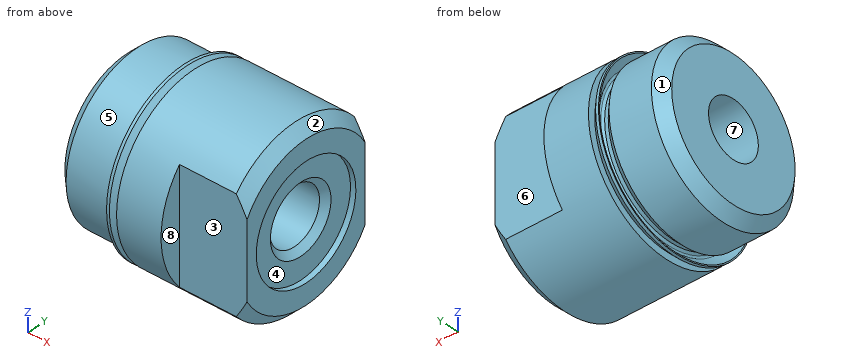
Autodesk Inventor part; units mm, degrees
ref_plane "cut1_XY" through (12.7, 4.699, 0) normal (1, 0, 0) x (0, 0, -1)
ref_plane "cut1_YZ" through (12.7, 4.699, 0) normal (0, 0, -1) x (0, 1, 0)
ref_plane "cut1_ZX" through (12.7, 4.699, 0) normal (0, 1, 0) x (1, 0, 0)
sketch "Sketch_1" plane through (0, 0, 0) normal (0, 0, 1) x (1, 0, 0)
  line L0 (12.7, 0) -> (0, 0)
  line L1 (0, 0) -> (0, 4.9085)
  line L2 (0, 4.9085) -> (0.762, 5.6706)
  line L3 (0.762, 5.6706) -> (3.7592, 5.6706)
  line L4 (3.7592, 5.6706) -> (4.2672, 5.1626)
  line L5 (4.2672, 5.1626) -> (4.7752, 5.1626)
  line L6 (4.7752, 5.1626) -> (4.7752, 6.1659)
  line L7 (4.7752, 6.1659) -> (11.938, 6.1659)
  line L8 (11.938, 6.1659) -> (12.7, 5.4039)
  line L9 (12.7, 5.4039) -> (12.7, 0)
  line L10 (12.7, 0) -> (0, 0)
revolve "Revolution1" add sketch "Sketch_1" angle 360 about axis through (12.7, 0, 0) along (1, 0, 0)
sketch "Sketch2" plane through (12.7, 0, 0) normal (1, 0, 0) x (0, 0, -1)
  point P0 (0, 0)
hole "Hole1" at (12.7, 0, 0) direction (-1, 0, 0) diameter 7.9248 depth 0.381
sketch "Sketch3" plane through (12.319, 0, 0) normal (1, 0, 0) x (0, 0, -1)
  point P0 (0, 0)
hole "Hole2" at (12.319, 0, 0) direction (-1, 0, 0) diameter 3.9624 depth 12.319 countersink diameter 4.826 countersink angle 90
sketch "Sketch_5" plane through (12.7, 0, 0) normal (1, 0, 0) x (0, 0, -1)
  line L0 (-24.6634, -12.3317) -> (24.6634, -12.3317)
  line L1 (24.6634, -12.3317) -> (24.6634, 12.3317)
  line L2 (24.6634, 12.3317) -> (-24.6634, 12.3317)
  line L3 (-24.6634, 12.3317) -> (-24.6634, -12.3317)
  line L4 (-12.3317, -4.699) -> (12.3317, -4.699)
  line L5 (12.3317, -4.699) -> (12.3317, 4.699)
  line L6 (12.3317, 4.699) -> (-12.3317, 4.699)
  line L7 (-12.3317, 4.699) -> (-12.3317, -4.699)
extrude "Extrusion1" cut sketch "Sketch_5" against normal blind 4.7752
sketch "Sketch_24" plane through (0, 0, 0) normal (0, 0, 1) x (1, 0, 0)
  line L0 (4.7752, 0) -> (4.2672, 0)
  line L1 (4.0665, 6.1659) -> (4.0665, 6.0817)
  line L2 (4.0665, 6.0817) -> (4.6636, 5.4846)
  arc A0 (4.6636, 5.305) -> (4.6636, 5.4846) centre (4.5738, 5.3948) ccw
  line L3 (4.6636, 5.305) -> (4.5212, 5.1626)
  line L4 (4.5212, 5.1626) -> (4.2672, 5.1626)
  line L5 (4.2672, 5.1626) -> (4.2672, 4.9085)
  line L6 (4.2672, 4.9085) -> (4.7752, 4.9085)
  line L7 (4.7752, 4.9085) -> (4.7752, 5.6603)
  line L8 (4.7752, 5.6603) -> (4.2697, 6.1659)
  line L9 (4.2697, 6.1659) -> (4.0665, 6.1659)
revolve "Revolution2" add sketch "Sketch_24" angle 360 about axis through (4.7752, 0, 0) along (1, 0, 0)
ref_plane "cut1_XY" through (12.7, 4.699, 0) normal (1, 0, 0) x (0, 0, -1)
ref_plane "cut1_YZ" through (12.7, 4.699, 0) normal (0, 0, -1) x (0, 1, 0)
ref_plane "cut1_ZX" through (12.7, 4.699, 0) normal (0, 1, 0) x (1, 0, 0)
ref_plane "cut2_XY" through (12.7, -4.699, 0) normal (1, 0, 0) x (0, 0, -1)
ref_plane "cut2_YZ" through (12.7, -4.699, 0) normal (0, 0, -1) x (0, 1, 0)
ref_plane "cut2_ZX" through (12.7, -4.699, 0) normal (0, 1, 0) x (1, 0, 0)
ref_plane "cutf1_XY" through (12.7, 0, 0) normal (0, 0, 1) x (1, 0, 0)
ref_plane "cutf1_YZ" through (12.7, 0, 0) normal (1, 0, 0) x (0, 1, 0)
ref_plane "cutf1_ZX" through (12.7, 0, 0) normal (0, 1, 0) x (0, 0, 1)
ref_plane "cutf2_XY" through (7.9248, 0, 0) normal (0, 0, 1) x (1, 0, 0)
ref_plane "cutf2_YZ" through (7.9248, 0, 0) normal (1, 0, 0) x (0, 1, 0)
ref_plane "cutf2_ZX" through (7.9248, 0, 0) normal (0, 1, 0) x (0, 0, 1)
ref_plane "lovra_XY" through (12.7, 0, 0) normal (1, 0, 0) x (0, 1, 0)
ref_plane "lovra_YZ" through (12.7, 0, 0) normal (0, 1, 0) x (0, 0, 1)
ref_plane "lovra_ZX" through (12.7, 0, 0) normal (0, 0, 1) x (1, 0, 0)
ref_plane "lovra1_XY" through (7.9248, 0, 0) normal (1, 0, 0) x (0, 0, -1)
ref_plane "lovra1_YZ" through (7.9248, 0, 0) normal (0, 0, -1) x (0, 1, 0)
ref_plane "lovra1_ZX" through (7.9248, 0, 0) normal (0, 1, 0) x (1, 0, 0)
ref_plane "lovra2_XY" through (7.9248, 4.699, 0) normal (1, 0, 0) x (0, 0, -1)
ref_plane "lovra2_YZ" through (7.9248, 4.699, 0) normal (0, 0, -1) x (0, 1, 0)
ref_plane "lovra2_ZX" through (7.9248, 4.699, 0) normal (0, 1, 0) x (1, 0, 0)
ref_plane "lovra21_XY" through (0, 0, 5.2705) normal (1, 0, 0) x (0, 0, -1)
ref_plane "lovra21_YZ" through (0, 0, 5.2705) normal (0, 0, -1) x (0, 1, 0)
ref_plane "lovra21_ZX" through (0, 0, 5.2705) normal (0, 1, 0) x (1, 0, 0)
ref_plane "lovra22_XY" through (0, 0, -5.2705) normal (1, 0, 0) x (0, 0, -1)
ref_plane "lovra22_YZ" through (0, 0, -5.2705) normal (0, 0, -1) x (0, 1, 0)
ref_plane "lovra22_ZX" through (0, 0, -5.2705) normal (0, 1, 0) x (1, 0, 0)
ref_plane "lovra3_XY" through (7.9248, -4.699, 0) normal (1, 0, 0) x (0, 0, -1)
ref_plane "lovra3_YZ" through (7.9248, -4.699, 0) normal (0, 0, -1) x (0, 1, 0)
ref_plane "lovra3_ZX" through (7.9248, -4.699, 0) normal (0, 1, 0) x (1, 0, 0)
ref_plane "olen_XY" through (12.7, 0, 0) normal (1, 0, 0) x (0, 0, -1)
ref_plane "olen_YZ" through (12.7, 0, 0) normal (0, 0, -1) x (0, 1, 0)
ref_plane "olen_ZX" through (12.7, 0, 0) normal (0, 1, 0) x (1, 0, 0)
ref_plane "to_mounting_bracket_XY" through (17.4752, 0, 0) normal (1, 0, 0) x (0, 0, -1)
ref_plane "to_mounting_bracket_YZ" through (17.4752, 0, 0) normal (0, 0, -1) x (0, 1, 0)
ref_plane "to_mounting_bracket_ZX" through (17.4752, 0, 0) normal (0, 1, 0) x (1, 0, 0)
ref_plane "to_nut_XY" through (0, 0, 0) normal (1, 0, 0) x (0, 0, -1)
ref_plane "to_nut_YZ" through (0, 0, 0) normal (0, 0, -1) x (0, 1, 0)
ref_plane "to_nut_ZX" through (0, 0, 0) normal (0, 1, 0) x (1, 0, 0)
ref_plane "to_pin_XY" through (23.8252, 0, 0) normal (0, 0, 1) x (1, 0, 0)
ref_plane "to_pin_YZ" through (23.8252, 0, 0) normal (1, 0, 0) x (0, 1, 0)
ref_plane "to_pin_ZX" through (23.8252, 0, 0) normal (0, 1, 0) x (0, 0, 1)
ref_plane "to_screw_XY" through (12.7, 0, 0) normal (0, 1, 0) x (1, 0, 0)
ref_plane "to_screw_YZ" through (12.7, 0, 0) normal (1, 0, 0) x (0, 0, -1)
ref_plane "to_screw_ZX" through (12.7, 0, 0) normal (0, 0, -1) x (0, 1, 0)
ref_plane "to_tube_XY" through (4.2672, 0, 0) normal (1, 0, 0) x (0, 0, -1)
ref_plane "to_tube_YZ" through (4.2672, 0, 0) normal (0, 0, -1) x (0, 1, 0)
ref_plane "to_tube_ZX" through (4.2672, 0, 0) normal (0, 1, 0) x (1, 0, 0)
properties part number "010000_rear_head"
Geometry check sheet. Reference: the model listing, model coordinates, mm. Face numbers are marked on the shaded views. A direction names the side the tool comes from. Give positions to 0.01 mm unless a question says otherwise; leave off trailing zeros. Order: outer loops, then holes, each group sorted by start corner. A loop starts at its lowest first (then second) coordinate and runs counter-clockwise, first axis right, second up. Notation, with made-up numbers: (68, 86.25) - (121, 86.25) arc R20 ccw to (121, 99.25) - close; hole circle Ø11 at (8.25, 56.25). An arc over 180 degrees is marked (long way). Answer as a JSON object with one key per item and string values.
(1) Cross-section at B-B (x = 5.75). Record the cut outline in (y, z).
Report:
{"outline": "circle Ø12.33 at (0, 0); hole circle Ø3.96 at (0, 0)"}
(2) Material ranges on line 1 (Y direction, x = 12.6, z = 0); line 2 (Y direction, x = 8.5, z = 0); line 3 (X direction, y = -2.25, z = -2.75), recorded low to high.
Report:
{"line 1": "-4.7 to -3.96, 3.96 to 4.7", "line 2": "-4.7 to -1.98, 1.98 to 4.7", "line 3": "0 to 12.32"}
(3) Depth check by flat-ended pin: pin 1 Ø3.5 at (y, z) = (-2, 1) entering from -X; pin 2 Ø3 at (x, y) = (1.5, 2) entering from -Z; pin 3 Ø1.2 at (y, z) = (-5.5, -0.5) entering from +X; pin 4 Ø1 at (y, z) = (-4.5, -4.5) entering from +X. Enter the tip coordinate at first touch or a pass-through.
Report:
{"pin 1": "x = 0", "pin 2": "z = -5.65", "pin 3": "x = 7.92", "pin 4": "x = 12.24"}
(4) Cross-section at C-C (x = 1.5). Record the cut outline in (y, z), then the cut area to 3 significant figures.
Report:
{"outline": "circle Ø11.34 at (0, 0); hole circle Ø3.96 at (0, 0)", "area": "88.7 mm^2"}
(5) Draft check along Z on the marked faces 1, 2, 3 and 4. Enter one of: released by +Z, released by -Z, zero draft, split by the parting line, or undercut.
Report:
{"face 1": "split by the parting line", "face 2": "released by +Z", "face 3": "zero draft", "face 4": "undercut"}
(6) Cross-section at A-A (x = 8.5). Record the cut outline in (y, z).
Report:
{"outline": "(-4.7, -3.99) arc R6.17 ccw to (4.7, -3.99) - (4.7, 3.99) arc R6.17 ccw to (-4.7, 3.99) - close; hole circle Ø3.96 at (0, 0)"}
(7) Tool access check on the marked faces 5, 6, 7 and 8. Record the directions out of +Z, -Z, +X, -X, +Y, -Y that give a thin tool (end or side, any length) a straight path to the whole face; none if there is none.
Report:
{"face 5": "-X", "face 6": "+Z, -Z, +X, +Y", "face 7": "+X, -X", "face 8": "+Z, -Z, +X, -Y"}
